Geometry check sheet. Reference: drawing and pictorial views, mm from the part's lowest x, y, z. A direction names the side the tool comes from. Give positions to 0.01 mm unless a question says otherwise; leave off trailing zeros. Order: outer loops, then holes, each group sorted by start corner. A loop starts at its lowest first (then second) coordinate and runs counter-clockwise, first axis right, second up.
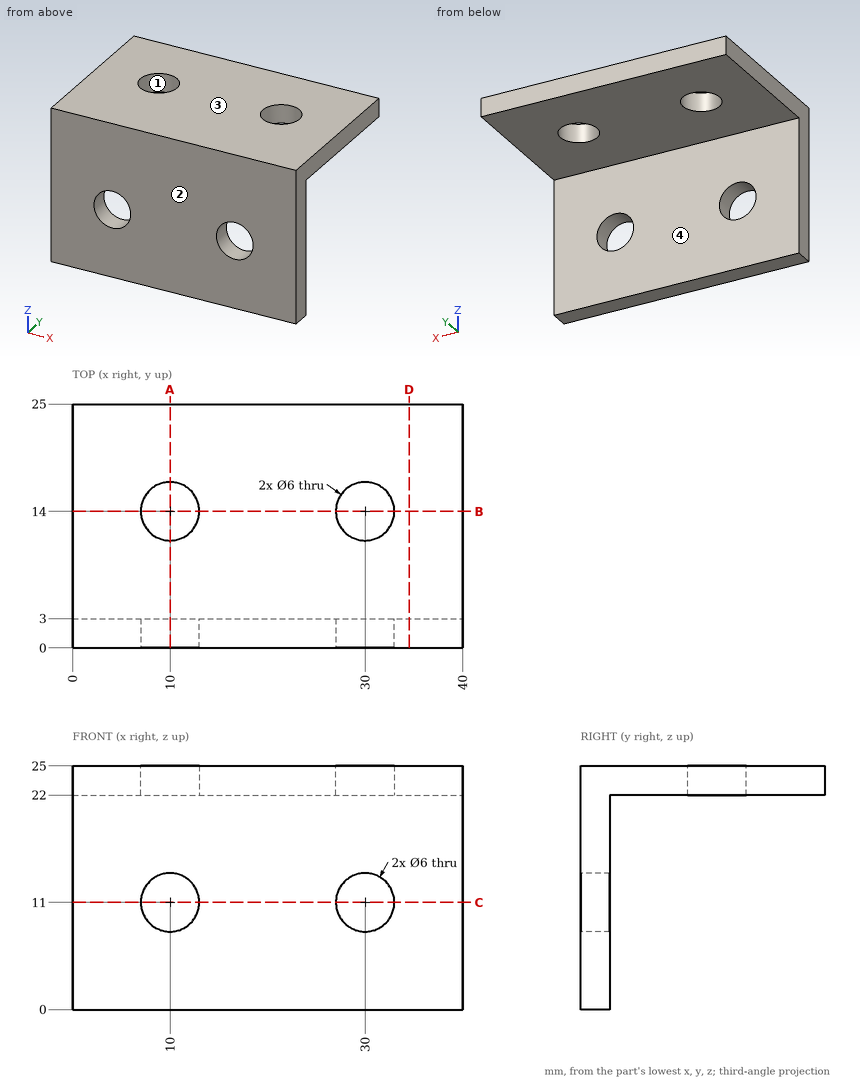
1) Section check A-A, the plane x = 10. Record the cut outline in (y, z).
Recorded:
outline: (0, 0) - (3, 0) - (3, 8) - (0, 8) - close; (0, 14) - (3, 14) - (3, 22) - (11, 22) - (11, 25) - (0, 25) - close; (17, 22) - (25, 22) - (25, 25) - (17, 25) - close
2) Material ranges on L1, parallel to Z at x = 30, y = 1.2; L2, parallel to Z at x = 14, y = 14.25; L3, parallel to Y at x = 10, z = 23.3, recorded low to high.
Recorded:
L1: z = 0 to 8, 14 to 25
L2: z = 22 to 25
L3: y = 0 to 11, 17 to 25
3) Section check D-D, the plane x = 34.5. Record the cut outline in (y, z).
Recorded:
outline: (0, 0) - (3, 0) - (3, 22) - (25, 22) - (25, 25) - (0, 25) - close
4) Section check B-B, the plane y = 14. Record the cut outline in (x, z), then the cut area to 3 significant figures.
Recorded:
outline: (0, 22) - (7, 22) - (7, 25) - (0, 25) - close; (13, 22) - (27, 22) - (27, 25) - (13, 25) - close; (33, 22) - (40, 22) - (40, 25) - (33, 25) - close
area: 84.0 mm2
5) Section check C-C, the plane z = 11. Record the cut outline in (x, y).
Recorded:
outline: (0, 0) - (7, 0) - (7, 3) - (0, 3) - close; (13, 0) - (27, 0) - (27, 3) - (13, 3) - close; (33, 0) - (40, 0) - (40, 3) - (33, 3) - close
6) Depth check by flat-ended pin: pin 1 Ø12 at (y, z) = (6.5, 17.5) entering from -X; pin 2 Ø1.5 at (x, y) = (25, 17.5) entering from -Z. Enter the tip coordinate at first touch or a pass-through.
Recorded:
pin 1: stops at x = 0
pin 2: stops at z = 22
7) Draft check along X on the marked faces 1 and 2. Enter one of: +X half, -X half, draft (parallel to the pull), parting line (faces both ways), or undercut.
Recorded:
face 1: undercut
face 2: draft
8) Set-up check for the marked faces 3 and 4: record each of +Z, -Z, +X, -X, +Y, -Y from which the full face is reachable in a straight line by a thin tool's end or side.
Recorded:
face 3: +Z, +X, -X, +Y, -Y
face 4: -Z, +X, -X, +Y
